Could you check a few things on this model? Use its own coordinates, in mm. Face numbers are marked on the shaded views. A direction names the side the tool comes from. Give positions to 0.01 mm unless a question says otherwise; leave off trailing zeros. Order: outer loops, then holes, each group sorted by start corner. A loop starts at its lowest first (then second) coordinate and runs counter-clockwise, first axis right, second up.
(1) Imagine slicing it at B-B, the plane x = 57. Write out the boundary of the cut face in (y, z), then the cut area to 3 significant figures.
(2) If we mould it in two halves opening along X, with no side actions, what happens to the marked faces 1, 2 and 3? For each: released by +X, released by -X, zero draft, split by the parting line, or undercut.
(3) Will these pins go through, and if not, where does the flat tip stop? pin 1 (1.6 mm diameter, centred on x = -74, y = 4, fed in from +Z); pin 2 (2 mm diameter, centred on x = -73.5, y = 4.5, fed in from -Z).
(4) On a 3-axis mill with a long thin cutter (end or side, diameter ignored), from which of +Z, -Z, +X, -X, +Y, -Y can I reach the whole of each face in a straight line? I mean the marked faces 4 and 5. Say none if no direction works.
(5) If I drill on probe 1 along Z at (x, y) = (51, 5.25); probe 2 along X at (y, z) = (7.5, 8.5); probe 3 along Y at (x, z) = (-39.5, -2.5), over which ranges is the centre line in solid material (lowest first)?
(6) Imagine slicing it at A-A, the plane x = -53.5. Write out the boundary of the cut face in (y, z), then the cut area to 3 significant figures.
(7) Imagine slicing it at C-C, the plane z = 0.5. Write out the boundary of the cut face in (x, y), then the cut area to 3 significant figures.
from build123d import *

# Parameters (mm, degrees)
SKETCH1_W           = 150
SKETCH1_H           = 35
SKETCH1_W_2         = 146
SKETCH1_H_2         = 31
SKETCH1_W_3         = 55
SKETCH1_H_3         = 25
BOSS_EXTRUDE1_DEPTH = 10
SKETCH2_W           = 55
SKETCH2_H           = 25
CUT_EXTRUDE3_DEPTH  = 8
SKETCH6_W           = 25
SKETCH6_H           = 5
CUT_EXTRUDE4_DEPTH  = 8
FILLET1_R           = 5


with BuildPart() as part:
    # Sketch1 → Boss-Extrude1 (new body)
    # profile 1 of 2: a face of its own
    with BuildSketch(Plane(origin=(0, 0, 0), x_dir=(1, 0, 0), z_dir=(0, 1, 0))):
        Rectangle(SKETCH1_W, SKETCH1_H)
        Rectangle(SKETCH1_W_2, SKETCH1_H_2, mode=Mode.SUBTRACT)
    # profile 2 of 2: a face of its own
    with BuildSketch(Plane(origin=(0, 0, 0), x_dir=(1, 0, 0), z_dir=(0, 1, 0))):
        with Locations((-45.5, 0)):
            Rectangle(SKETCH1_W_3, SKETCH1_H_3)
    extrude(amount=BOSS_EXTRUDE1_DEPTH)

    # Sketch2 → Cut-Extrude3 (cut)
    with BuildSketch(Plane(origin=(0, 10, 0), x_dir=(1, 0, 0), z_dir=(0, 1, 0))):
        with Locations((-45.5, 0)):
            Rectangle(SKETCH2_W, SKETCH2_H)
    extrude(amount=-CUT_EXTRUDE3_DEPTH, mode=Mode.SUBTRACT)

    # Sketch6 → Cut-Extrude4 (cut)
    with BuildSketch(Plane.ZY.offset(75)):
        with Locations((0, 4.5)):
            Rectangle(SKETCH6_W, SKETCH6_H)
    extrude(amount=-CUT_EXTRUDE4_DEPTH, mode=Mode.SUBTRACT)

    # Fillet1
    fillet1_edges = [part.edges().sort_by_distance(p)[0] for p in [
        (-75, 5, 17.5),
        (-75, 5, -17.5),
        (75, 5, -17.5),
        (75, 5, 17.5),
    ]]
    fillet(fillet1_edges, radius=FILLET1_R - 0.0001)  # a hair under: the kernel refuses the full size


solid = part.part
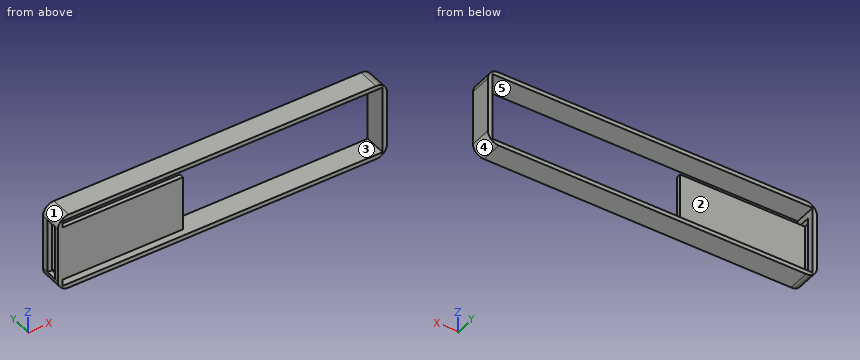
Answer block:
1. outline: (0, -17.5) - (10, -17.5) - (10, -15.5) - (0, -15.5) - close; (0, 15.5) - (10, 15.5) - (10, 17.5) - (0, 17.5) - close
1. area: 40.0 mm2
2. face 1: released by -X
2. face 2: zero draft
2. face 3: undercut
3. pin 1: stops at z = 16.34
3. pin 2: stops at z = -16.83
4. face 4: -Z, +X, +Y, -Y
4. face 5: +Y, -Y
5. probe 1: z = -17.5 to -15.5, 15.5 to 17.5
5. probe 2: x = -75 to -73, 73 to 75
5. probe 3: y = 0 to 2
6. outline: (0, -17.5) - (10, -17.5) - (10, -15.5) - (0, -15.5) - close; (0, -12.5) - (2, -12.5) - (2, 12.5) - (0, 12.5) - close; (0, 15.5) - (10, 15.5) - (10, 17.5) - (0, 17.5) - close
6. area: 90.0 mm2
7. outline: (-75, 0) - (-18, 0) - (-18, 2) - (-75, 2) - close; (-75, 7) - (-73, 7) - (-73, 10) - (-75, 10) - close; (73, 0) - (75, 0) - (75, 10) - (73, 10) - close
7. area: 140 mm2
